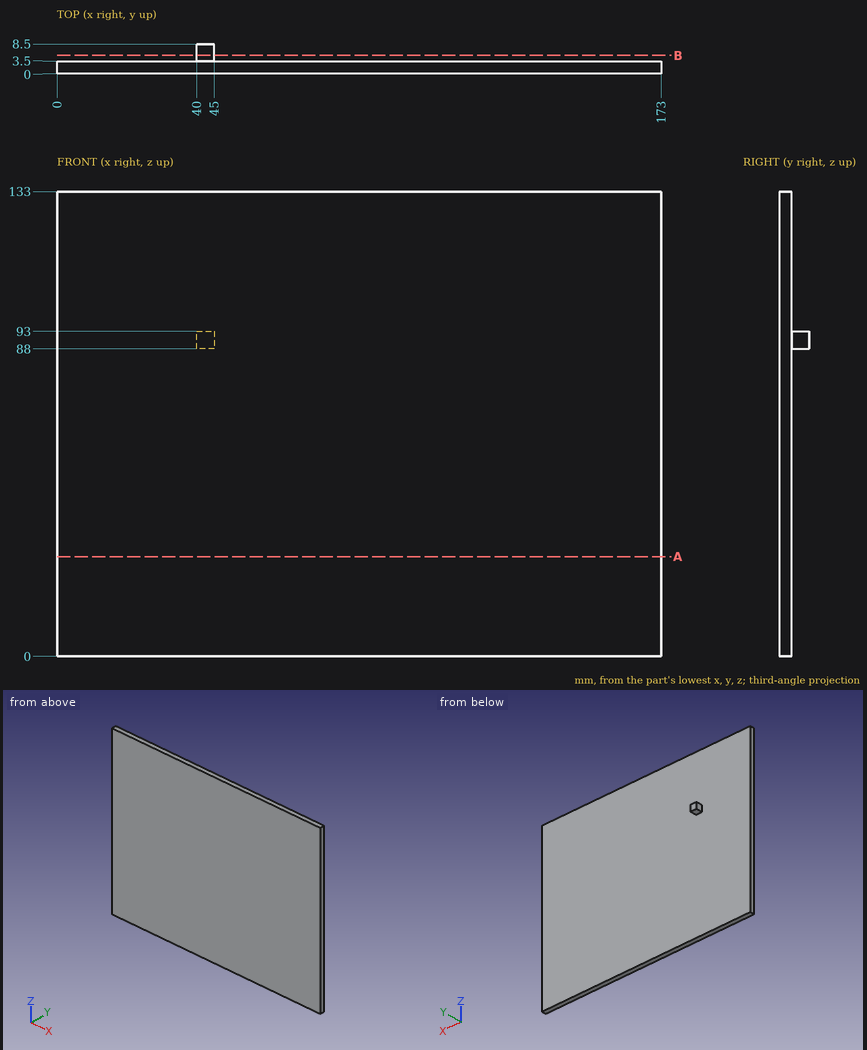
Study the drawing (mm; zero at the part's minimum x, y, z) and answer. Give positions to 0.01 mm unless a question says otherwise; leave off trailing zeros. Loops run counter-clockwise (first coordinate to the right, second up) from the corner with the lowest first, then second, coordinate; pieces in that order, holes last. Notation, with made-up numbers: (54, 51) -> (60, 51) arc R13 ccw to (60, 60) -> close; hole circle Ø6 at (-26, 15). An arc over 180 degrees is marked (long way). Write item = value, one per line. Start each with the question number.
(1) Given pin 1 Ø1.5 at (y, z) = (7, 90) entering from -X; pin 2 Ø1.5 at (x, z) = (88.5, 85) entering from +Y; pin 3 Ø4 at (x, y) = (43.5, 6) entering from -Z, each flat-ended and moving along its own axis, determine where each tip first touches the part or whether it passes through.
(2) Find section A-A on z = 28.5. Give the vertices of the cut face in (x, y), and give its area (4 significant figures).
(3) Find section B-B on y = 5.25. Give the vertices of the cut face in (x, z).
(4) Find the intervals of material crossed by probe 1 along Y at (x, z) = (142, 52); probe 2 along Z at (x, y) = (43.5, 4.75), in increasing order. Write a range as from..to.
From the geometry:
q1.pin_1 = 40
q1.pin_2 = 3.5
q1.pin_3 = 88
q2.outline = (0, 0) -> (173, 0) -> (173, 3.5) -> (0, 3.5) -> close
q2.area = 605.5 mm^2
q3.outline = (40, 88) -> (45, 88) -> (45, 93) -> (40, 93) -> close
q4.probe_1 = 0..3.5
q4.probe_2 = 88..93
